Design review of the part built by this model. Coordinates are the model's own, in mm. A direction names the side the tool comes from. Coordinates: 2 decimals unless noted, no trailing zeros. Loops run counter-clockwise (first coordinate to the right, second up) from the corner with the lowest first, then second, coordinate; pieces in that order, holes last. Notation, with made-up numbers: (-19.75, 80.5) - (18.25, 80.5) arc R25 cw to (18.25, 119.5) - close; hole circle Ø2 at (-0.5, 44). An arc over 180 degrees is marked (long way). Use one line per item in the form item = value. Start each with the question number.
(1) For L1, parallel to Z at x = 32, y = 18; L2, parallel to Z at x = 20, y = 1; L3, parallel to Y at x = 25, z = 14.5, list the stretches that pass through material, from the lowest coordinate up.
(2) Clearance check with flat-ended pins moving along their axes: pin 1 Ø7 at (x, y) = (27.5, 13) entering from +Z; pin 2 Ø12 at (x, y) = (11.5, 8.5) entering from -Z; pin 3 Ø1.5 at (x, y) = (8.5, 9.5) entering from -Z. State where each tip first meets the part, or that it passes through.
(3) Tool access review of faces 1 (the face through (19.7, 27.1, 41.7)), 2 (the face through (19.72, 24.3, 19.52)), 3 (the face through (19.72, 22.324, 16.692)), 4 (the face through (20, 11, 20)): name each direction out of +Z, -Z, +X, -X, +Y, -Y from which nothing blocks a thin tool from reaching the whole face with its end or side.
(4) Add section C-C (x = 14.5). State the section outline as (y, z) points.
(5) The part is to be moulded in two halves that separate along Z. For faces 5 (the face through (19.72, 0, 10.14)), 6 (the face through (19.72, 29.04, 24.76)), 7 (the face through (19.7, 34, 15.1)), say which applies: pulls with the +Z half, pulls with the -Z half, needs draft (parallel to the pull), parting line crosses it, or undercut.
(6) Add section D-D (y = 17.5). State the section outline as (x, z) points, plus the area to 3 significant figures.
(7) Add section A-A (z = 8). State the section outline as (x, y) points.
(8) Add section B-B (x = 20). State the section outline as (y, z) points.
```python
from build123d import *

# Parameters (mm, degrees)
F1_DEPTH = 40
F2_R     = 2
F3_DEPTH = 9.6
F4_SIZE  = 2


with BuildPart() as f1:
    # F0 (on Right) → F1 (new body)
    with BuildSketch(Plane.YZ):
        with BuildLine():
            Line((0, 20), (0, 0))
            ThreePointArc((0, 0), (2.12132, 0.87868), (3, 3))
            Line((3, 3), (3, 17))
            Line((3, 17), (21, 17))
            ThreePointArc((21, 17), (22.341641, 16.683282), (23.4, 15.8))
            ThreePointArc((23.4, 15.8), (34.164312, 15.27455), (32.687463, 25.95001))
            ThreePointArc((32.687463, 25.95001), (31.712786, 26.927793), (31.279221, 28.238547))
            Line((31.279221, 28.238547), (28.514858, 59.835355))
            ThreePointArc((28.514858, 59.835355), (26.485898, 58.771775), (25.799112, 56.586321))
            Line((25.799112, 56.586321), (28.448779, 26.300488))
            ThreePointArc((28.448779, 26.300488), (29.051308, 24.74351), (30.392779, 23.749689))
            ThreePointArc((30.392779, 23.749689), (31.949109, 17.297639), (25.385968, 18.285714))
            ThreePointArc((25.385968, 18.285714), (24.279012, 19.535463), (22.675445, 20))
            Line((22.675445, 20), (0, 20))
        make_face()
    extrude(amount=F1_DEPTH)

    # F2 (on face) → F3 (cut)
    with BuildSketch(Plane(origin=(0, 3, 0), x_dir=(-1, 0, 0), z_dir=(0, 1, 0))):
        with Locations((-20, 8)):
            Circle(F2_R)
    extrude(amount=-F3_DEPTH, mode=Mode.SUBTRACT)

    # F4
    f4_edges = [f1.edges().sort_by_distance(p)[0] for p in [
        (20, 3, 17),
    ]]
    chamfer(f4_edges, length=F4_SIZE)


solid = f1.part
```
Computed values:
q1.L1 = 17 to 20
q1.L2 = 0.17 to 6, 10 to 20
q1.L3 = 0 to 3, 24.67 to 33.33
q2.pin_1 = 20
q2.pin_2 = 1.34
q2.pin_3 = 17
q3.face_1 = +X, -X, -Y
q3.face_2 = +Z, +X, -X
q3.face_3 = -Z, +X, -X
q3.face_4 = +Z, +X, -X, -Y
q4.outline = (0, 0) arc R3 ccw to (3, 3) - (3, 15) - (5, 17) - (21, 17) arc R3 cw to (23.4, 15.8) arc R7 ccw (long way) to (32.69, 25.95) arc R3 cw to (31.28, 28.24) - (28.51, 59.84) arc R3 ccw to (25.8, 56.59) - (28.45, 26.3) arc R3 ccw to (30.39, 23.75) arc R4 cw (long way) to (25.39, 18.29) arc R3 ccw to (22.68, 20) - (0, 20) - close
q5.face_5 = needs draft
q5.face_6 = undercut
q5.face_7 = parting line crosses it
q6.outline = (0, 17) - (40, 17) - (40, 20) - (0, 20) - close
q6.area = 120 mm^2
q7.outline = (0, 0) - (18, 0) - (18, 3) - (0, 3) - close; (22, 0) - (40, 0) - (40, 3) - (22, 3) - close
q8.outline = (0, 0) arc R3 ccw to (3, 3) - (3, 6) - (0, 6) - close; (0, 10) - (3, 10) - (3, 15) - (5, 17) - (21, 17) arc R3 cw to (23.4, 15.8) arc R7 ccw (long way) to (32.69, 25.95) arc R3 cw to (31.28, 28.24) - (28.51, 59.84) arc R3 ccw to (25.8, 56.59) - (28.45, 26.3) arc R3 ccw to (30.39, 23.75) arc R4 cw (long way) to (25.39, 18.29) arc R3 ccw to (22.68, 20) - (0, 20) - close
